Design review of the part built by this model. Coordinates are the model's own, in mm. A direction names the side the tool comes from. Round coordinates to 2 decimals unless told otherwise and drop trailing zeros. Loops run counter-clockwise (first coordinate to the right, second up) from the corner with the lowest first, then second, coordinate; pieces in that order, holes last. Notation, with made-up numbers: M -20.5,30.5 L 8.5,30.5 A19 ccw 8.5,53.5 Z; hole C -21.5,70 d4. An arc over 180 degrees is marked long. Use a Markdown table: item, result.
from build123d import *

# Parameters (mm, degrees)
SKETCH_W        = 36
SKETCH_H        = 36
PAD_DEPTH       = 25
SKETCH001_W     = 30.4
SKETCH001_H     = 30.4
POCKET_DEPTH    = 22
SKETCH002_R     = 4
PAD001_DEPTH    = 6
SKETCH003_R     = 1
POCKET001_DEPTH = 6
SKETCH004_W     = 4
SKETCH004_H     = 25
PAD002_DEPTH    = 32
SKETCH005_W     = 4
SKETCH005_H     = 25
PAD003_DEPTH    = 32
SKETCH006_W     = 70
SKETCH006_H     = 25
PAD004_DEPTH    = 4
SKETCH007_W     = 70
SKETCH007_H     = 25
PAD005_DEPTH    = 4
PAD006_DEPTH    = 25
PAD007_DEPTH    = 25
SKETCH010_W     = 20
SKETCH010_H     = 50
PAD008_DEPTH    = 4
SKETCH011_W     = 20
SKETCH011_H     = 50
PAD009_DEPTH    = 4
SKETCH012_R     = 2.1
POCKET002_DEPTH = 120
PAD010_DEPTH    = 4
PAD011_DEPTH    = 4


with BuildPart() as part:
    # Sketch → Pad (new body)
    with BuildSketch(Plane.XY):
        Rectangle(SKETCH_W, SKETCH_H)
    extrude(amount=PAD_DEPTH)

    # Sketch001 (on Face6 of Pad) → Pocket (cut)
    with BuildSketch(Plane.XY.offset(25)):
        Rectangle(SKETCH001_W, SKETCH001_H)
    extrude(amount=-POCKET_DEPTH, mode=Mode.SUBTRACT)

    # Sketch002 (on Face11 of Pocket) → Pad001 (join)
    with BuildSketch(Plane.XY.offset(3)):
        with Locations((-14, 14)):
            Circle(SKETCH002_R)
        with Locations((14, 14)):
            Circle(SKETCH002_R)
        with Locations((14, -14)):
            Circle(SKETCH002_R)
        with Locations((-14, -14)):
            Circle(SKETCH002_R)
    extrude(amount=PAD001_DEPTH)

    # Sketch003 (on DatumPlane) → Pocket001 (cut)
    with BuildSketch(Plane.XY.offset(9)):
        with Locations((-14, -14)):
            Circle(SKETCH003_R)
        with Locations((14, -14)):
            Circle(SKETCH003_R)
        with Locations((14, 14)):
            Circle(SKETCH003_R)
        with Locations((-14, 14)):
            Circle(SKETCH003_R)
    extrude(amount=-POCKET001_DEPTH, mode=Mode.SUBTRACT)

    # Sketch004 (on DatumPlane) → Pad002 (join)
    with BuildSketch(Plane.YZ.offset(18)):
        with Locations((0, 12.5)):
            Rectangle(SKETCH004_W, SKETCH004_H)
    extrude(amount=PAD002_DEPTH)

    # Sketch005 (on DatumPlane) → Pad003 (join)
    with BuildSketch(Plane(origin=(-18, 0, 0), x_dir=(0, -1, 0), z_dir=(-1, 0, 0))):
        with Locations((0, 12.5)):
            Rectangle(SKETCH005_W, SKETCH005_H)
    extrude(amount=PAD003_DEPTH)

    # Sketch006 (on DatumPlane) → Pad004 (join)
    with BuildSketch(Plane(origin=(-50, 0, 0), x_dir=(0, -1, 0), z_dir=(-1, 0, 0))):
        with Locations((33, 12.5)):
            Rectangle(SKETCH006_W, SKETCH006_H)
    extrude(amount=PAD004_DEPTH)

    # Sketch007 (on DatumPlane) → Pad005 (join)
    with BuildSketch(Plane.YZ.offset(50)):
        with Locations((-33, 12.5)):
            Rectangle(SKETCH007_W, SKETCH007_H)
    extrude(amount=PAD005_DEPTH)

    # Sketch008 (on DatumPlane) → Pad006 (join)
    with BuildSketch(Plane(origin=(0, 0, 0), x_dir=(1, 0, 0), z_dir=(0, 0, -1))):
        Polygon((18, 18), (18, 2), (35, 2), align=None)
        Polygon((18, -2), (18, -18), (35, -2), align=None)
        Polygon((-18, -18), (-18, -2), (-35, -2), align=None)
        Polygon((-18, 2), (-18, 18), (-35, 2), align=None)
    extrude(amount=-PAD006_DEPTH)

    # Sketch009 (on DatumPlane) → Pad007 (join)
    with BuildSketch(Plane(origin=(0, 0, 0), x_dir=(1, 0, 0), z_dir=(0, 0, -1))):
        Polygon((50, 2), (50, 8), (44, 2), align=None)
        Polygon((-50, 2), (-44, 2), (-50, 8), align=None)
    extrude(amount=-PAD007_DEPTH)

    # Sketch010 (on DatumPlane) → Pad008 (join)
    with BuildSketch(Plane.YZ.offset(54)):
        with Locations((-58, 12.5)):
            Rectangle(SKETCH010_W, SKETCH010_H)
    extrude(amount=-PAD008_DEPTH)

    # Sketch011 (on DatumPlane) → Pad009 (join)
    with BuildSketch(Plane(origin=(-54, 0, 0), x_dir=(0, -1, 0), z_dir=(-1, 0, 0))):
        with Locations((58, 12.5)):
            Rectangle(SKETCH011_W, SKETCH011_H)
    extrude(amount=-PAD009_DEPTH)

    # Sketch012 (on DatumPlane) → Pocket002 (cut)
    with BuildSketch(Plane.YZ.offset(54)):
        with Locations((-58, 29.488935)):
            Circle(SKETCH012_R)
        with Locations((-58, 12.488935)):
            Circle(SKETCH012_R)
        with Locations((-58.000031, -4.511065)):
            Circle(SKETCH012_R)
    extrude(amount=-POCKET002_DEPTH, mode=Mode.SUBTRACT)

    # Sketch013 (on DatumPlane) → Pad010 (join)
    with BuildSketch(Plane.YZ.offset(54)):
        Polygon((-48, 25.003424), (-48, 37.443424), (-37, 25.003424), align=None)
        Polygon((-48, 0), (-48, -12.489775), (-37, 0), align=None)
    extrude(amount=-PAD010_DEPTH)

    # Sketch014 (on DatumPlane) → Pad011 (join)
    with BuildSketch(Plane.YZ.offset(-50)):
        Polygon((-47.989925, 24.913122), (-47.989925, 37.485035), (-37.0298, 24.913122), align=None)
        Polygon((-47.989925, -12.480257), (-47.989925, 0), (-37.0298, 0), align=None)
    extrude(amount=-PAD011_DEPTH)


solid = part.part
1. Take a section at A-A on y = -32. Give the boundary of the cut face in (x, z), and give its area (3 significant figures).
Check values:
| item | result |
|---|---|
| outline | M -54,0 L -50,0 L -50,25 L -54,25 Z; M 50,0 L 54,0 L 54,25 L 50,25 Z |
| area | 200 mm² |
2. Machinability: for faces 1 (the face through (47, -5, 12)), 2 (the face through (13, -13, 9)), 3 (the face through (44, 2, 12)), which of the approach directions +Z, -Z, +X, -X, +Y, -Y give a long, thin tool a straight path to every point of the face, cutting with its end or side? Answer none if there is none.
Check values:
| item | result |
|---|---|
| face 1 | +Z, -Z, -Y |
| face 2 | +Z |
| face 3 | +Z, -Z, +X, +Y |
3. Take a section at B-B on z = 16.5. Give the boundary of the cut face in (x, y).
Check values:
| item | result |
|---|---|
| outline | M -54,-68 L -50,-68 L -50,-8 L -44,-2 L -35,-2 L -18,-18 L 18,-18 L 35,-2 L 44,-2 L 50,-8 L 50,-68 L 54,-68 L 54,2 L 35,2 L 18,18 L -18,18 L -35,2 L -54,2 Z; hole M -15.2,-15.2 L 15.2,-15.2 L 15.2,15.2 L -15.2,15.2 Z |
4. Wall thickness on line 1 along Y through (x, z) = (-14, 5.95); line 2 along Z through (x, y) = (-51, -58); line 3 along Y through (x, z) = (4, 24.5): over which ranges is each line inside the solid? List them lowest first. Write a range as from..to.
Check values:
| item | result |
|---|---|
| line 1 | y = -18..-15, -13..-10, 10..13, 15..18 |
| line 2 | z = -12.5..-6.61, -2.41..10.39, 14.59..27.39, 31.59..37.5 |
| line 3 | y = -18..-15.2, 15.2..18 |
5. Take a section at C-C on y = -58. Count the separate pieces of the cut face and the enclosed holes in it, and give its area (3 significant figures).
Check values:
| item | result |
|---|---|
| separate pieces | 8 |
| enclosed holes | 0 |
| area | 299 mm² |
6. Insertion check: pin 1 (1.2 mm diameter, centred on x = 51, y = -45, fed in from -Z); pin 2 (4 mm diameter, centred on x = 3.5, z = 2.5, fed in from -Y); pin 3 (8 mm diameter, centred on x = -26, z = 21, fed in from +Y); pin 4 (10 mm diameter, centred on x = -42.5, y = -24, fed in from +Z). Each pin has a flat end and moves straight along its axis. Give the tip position at first contact, or say it passes through.
Check values:
| item | result |
|---|---|
| pin 1 | stops at z = -9.76 |
| pin 2 | stops at y = -18 |
| pin 3 | stops at y = 14.24 |
| pin 4 | passes through |
7. The part is to be moulded in two halves that separate along X. For faces 4 (the face through (54, -41, 13)), 5 (the face through (0, -6, 0)), 6 (the face through (-39, -2, 12)), 7 (the face through (-47, -5, 12)), say which applies: pulls with the +X half, pulls with the -X half, needs draft (parallel to the pull), parting line crosses it, or undercut.
Check values:
| item | result |
|---|---|
| face 4 | pulls with the +X half |
| face 5 | needs draft |
| face 6 | undercut |
| face 7 | undercut |
8. Take a section at D-D on x = -0.5. Give the boundary of the cut face in (y, z).
Check values:
| item | result |
|---|---|
| outline | M -18,0 L 18,0 L 18,25 L 15.2,25 L 15.2,3 L -15.2,3 L -15.2,25 L -18,25 Z |
